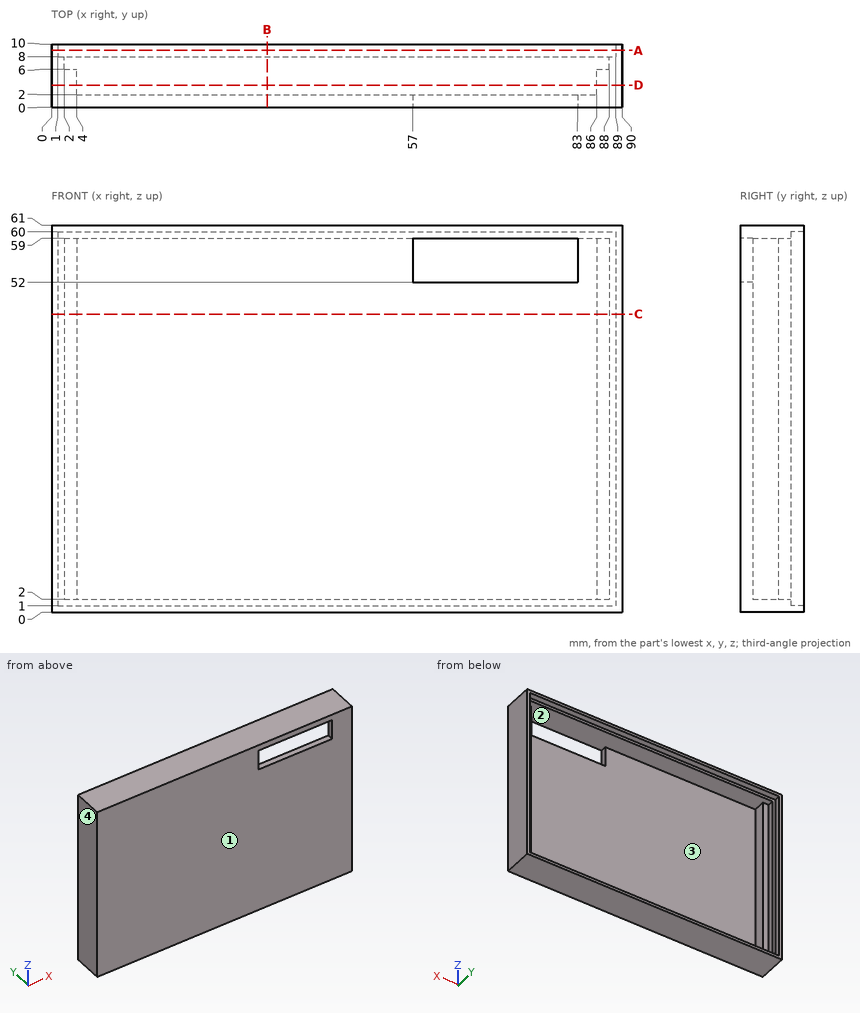
Drawing for the job (mm, zero at the part's lowest x, y, z). Round coordinates to 2 decimals unless told otherwise and drop trailing zeros. Order: outer loops, then holes, each group sorted by start corner. A loop starts at its lowest first (then second) coordinate and runs counter-clockwise, first axis right, second up.
Item 1: Probe line 1 along X through (y, z) = (4, 24.5); line 2 along X through (y, z) = (9, 22); line 3 along Z through (x, y) = (55.5, 4). List the from-to ranges inside material, lowest first.
Item 2: Pin check, flat tips, straight feed: pin 1 (2 mm diameter, centred on y = 4, z = 28, fed in from -X); pin 2 (1 mm diameter, centred on x = 87, z = 18.5, fed in from +Y). Stop position of each tip, or through.
Item 3: Saw through at D-D on y = 3.5. Write the cut outline in (x, z), then the cut area to 3 significant figures.
Item 4: Saw through at C-C on z = 47. Write the cut outline in (x, y), then the cut area to 3 significant figures.
Item 5: Saw through at B-B on x = 34. Write the cut outline in (y, z).
Item 6: Saw through at A-A on y = 9. Write the cut outline in (x, z), then the cut area to 3 significant figures.
Item 7: Mould opens along X. For the marked faces 1, 2, 3 and 4 say: pulls with the +X half, pulls with the -X half, needs draft (parallel to the pull), parting line crosses it, or undercut.
Reported:
1. line 1: x = 0 to 4, 86 to 90
1. line 2: x = 0 to 1, 89 to 90
1. line 3: z = 0 to 2, 59 to 61
2. pin 1: stops at x = 0
2. pin 2: stops at y = 6
3. outline: (0, 0) - (90, 0) - (90, 61) - (0, 61) - close; hole (4, 2) - (86, 2) - (86, 59) - (4, 59) - close
3. area: 816 mm2
4. outline: (0, 0) - (90, 0) - (90, 10) - (89, 10) - (89, 8) - (88, 8) - (88, 6) - (86, 6) - (86, 2) - (4, 2) - (4, 6) - (2, 6) - (2, 8) - (1, 8) - (1, 10) - (0, 10) - close
4. area: 224 mm2
5. outline: (0, 0) - (10, 0) - (10, 1) - (8, 1) - (8, 2) - (2, 2) - (2, 59) - (8, 59) - (8, 60) - (10, 60) - (10, 61) - (0, 61) - close
6. outline: (0, 0) - (90, 0) - (90, 61) - (0, 61) - close; hole (1, 1) - (89, 1) - (89, 60) - (1, 60) - close
6. area: 298 mm2
7. face 1: needs draft
7. face 2: undercut
7. face 3: undercut
7. face 4: pulls with the -X half
